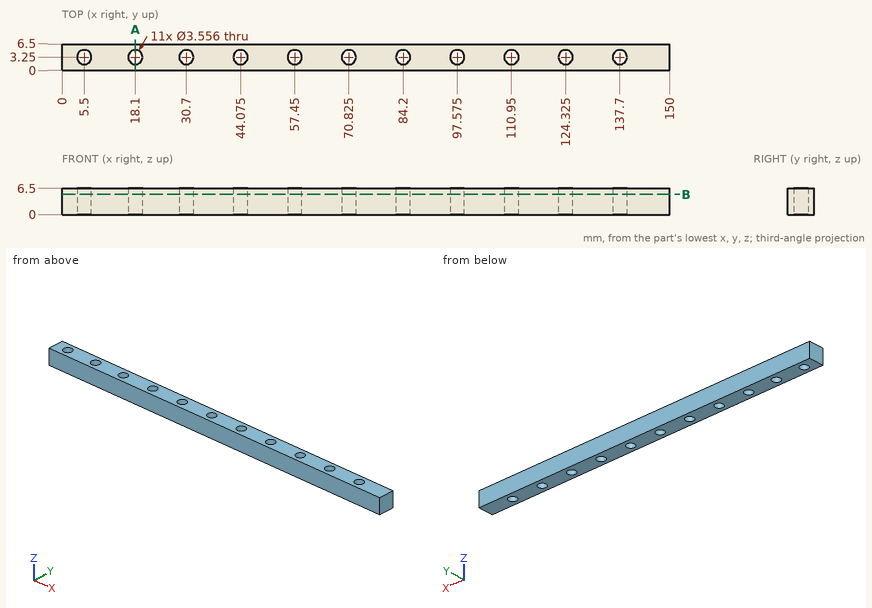
Source: three-view drawing plus pictorial views. Frame: mm from the lowest corner of the part. Round coordinates to 2 decimals unless told otherwise and drop trailing zeros. Write each loop counter-clockwise with the first axis right and the second up, starting at its lowest first coordinate (ties: lowest second). Pieces come first, ordered by that corner, then holes. Notation, with made-up numbers: M 43.25,73.25 L 76.25,73.25 A20 ccw 76.25,100.25 Z; hole C 67.5,-25.5 d10. An arc over 180 degrees is marked long. Write item = value, one per line.
Item 1: Material intervals for line 1 along Y through (x, z) = (124.5, 5); line 2 along Y through (x, z) = (138.5, 2.75), sorted ascending. Write a range as [from, to].
Findings:
line_1 = [0, 1.48], [5.02, 6.5]
line_2 = [0, 1.66], [4.84, 6.5]
Item 2: Section query A-A on x = 18.1. Return loops of the section in (y, z), then the cut area to 3 significant figures.
Findings:
outline = M 0,0 L 1.47,0 L 1.47,6.5 L 0,6.5 Z; M 5.03,0 L 6.5,0 L 6.5,6.5 L 5.03,6.5 Z
area = 19.1 mm^2
Item 3: Section query B-B on z = 5. State how many separate pieces and enclosed holes the cut face has, then the cut area to 3 significant figures.
Findings:
separate_pieces = 1
enclosed_holes = 11
area = 866 mm^2
